Answer from the drawing. Dimensions are ordinates in mm from the lowest x, y and z of the part. Give positions to 0.01 mm unless a question says otherwise; leave off trailing zeros. Write each loop counter-clockwise with the first axis right and the second up, starting at its lowest first coordinate (ties: lowest second). Pieces come first, ordered by that corner, then holes.
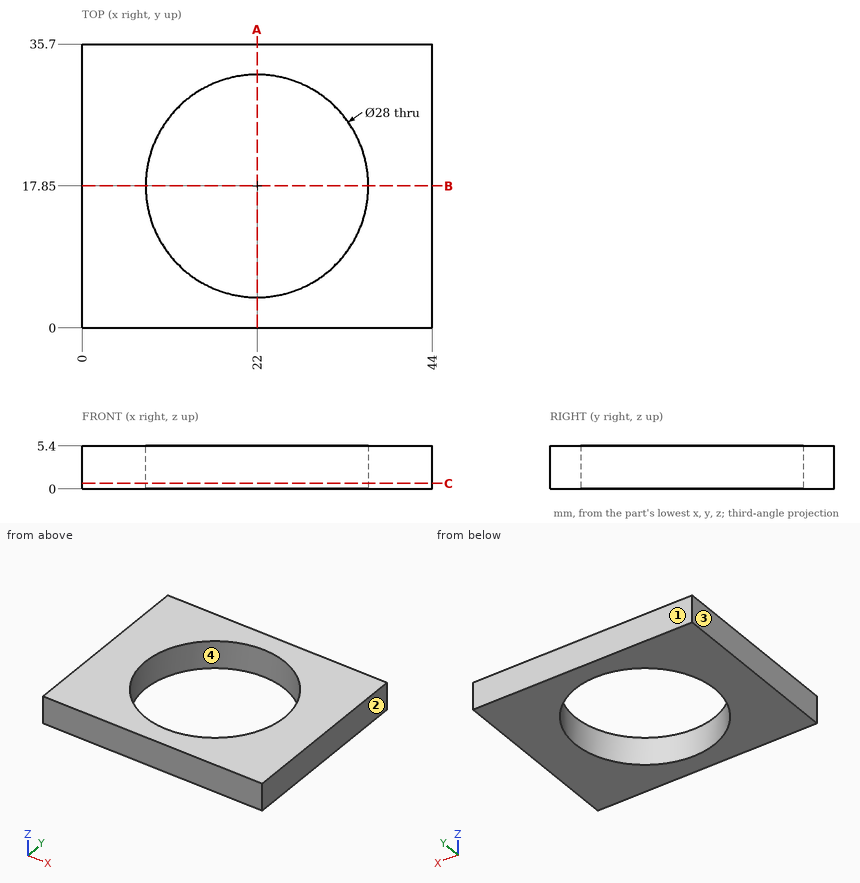
Item 1: Determine the mould class of the marked faces 1, 2, 3 and 4 for opening direction X: pulls with the +X half, pulls with the -X half, needs draft (parallel to the pull), parting line crosses it, or undercut.
Conclusion:
face 1: needs draft
face 2: pulls with the +X half
face 3: pulls with the -X half
face 4: undercut
Item 2: A cutting plane is placed at C-C, the plane z = 0.7. Give the vertices of the cut face in (x, y).
Conclusion:
outline: (0, 0) - (44, 0) - (44, 35.7) - (0, 35.7) - close; hole circle Ø28 at (22, 17.85)
Item 3: A cutting plane is placed at A-A, the plane x = 22. Give the vertices of the cut face in (y, z), plus the area to 3 significant figures.
Conclusion:
outline: (0, 0) - (3.85, 0) - (3.85, 5.4) - (0, 5.4) - close; (31.85, 0) - (35.7, 0) - (35.7, 5.4) - (31.85, 5.4) - close
area: 41.6 mm2
Item 4: Consider probe 1 along X at (y, z) = (17.85, 4.25); probe 2 along Y at (x, z) = (22, 2.5); probe 3 along Y at (x, z) = (12.5, 1.1). Determine where each line is inside the solid, lowest interval first.
Conclusion:
probe 1: x = 0 to 8, 36 to 44
probe 2: y = 0 to 3.85, 31.85 to 35.7
probe 3: y = 0 to 7.57, 28.13 to 35.7
Item 5: This flat-tipped pin is pushed along its axis until it touches: P1, Ø5, axis at x = 16.5, y = 27.5, coming from the +Z side. Where does it stop, or does it pass through?
Conclusion:
P1: passes through
Item 6: A cutting plane is placed at B-B, the plane y = 17.85. Give the vertices of the cut face in (x, z).
Conclusion:
outline: (0, 0) - (8, 0) - (8, 5.4) - (0, 5.4) - close; (36, 0) - (44, 0) - (44, 5.4) - (36, 5.4) - close
